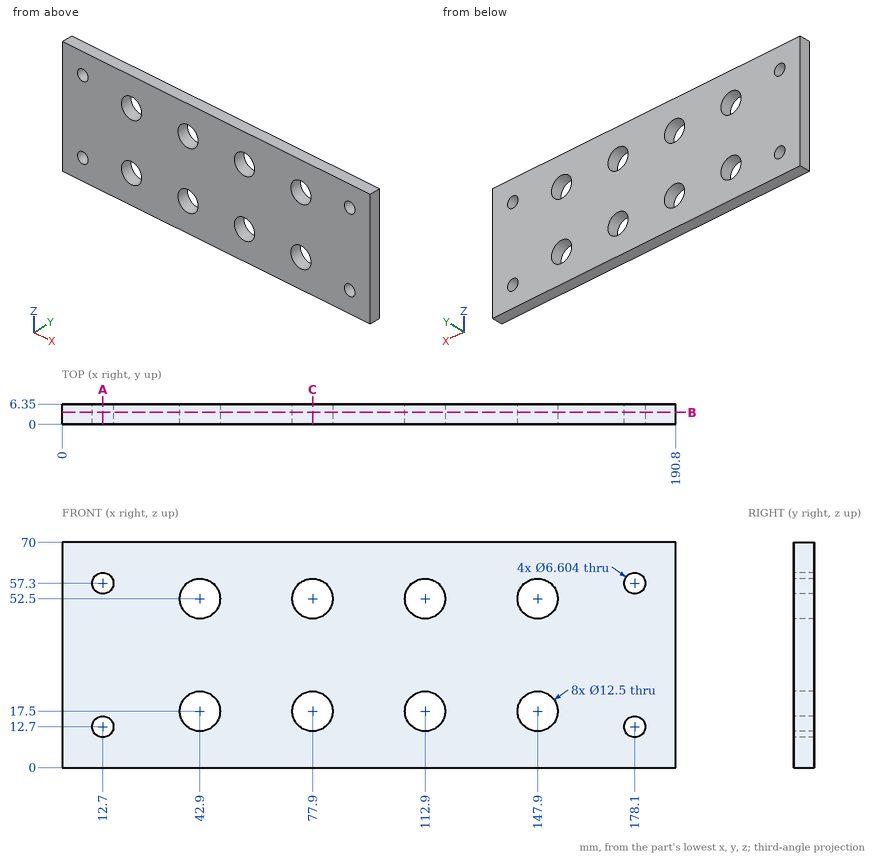
Geometry check sheet. Reference: drawing and pictorial views, mm from the part's lowest x, y, z. Round coordinates to 2 decimals unless told otherwise and drop trailing zeros. Loops run counter-clockwise (first coordinate to the right, second up) from the corner with the lowest first, then second, coordinate; pieces in that order, holes last. Notation, with made-up numbers: (86.5, 50) - (99.5, 50) arc R24 ccw to (99.5, 87) - close; hole circle Ø7 at (52.25, 38). An arc over 180 degrees is marked (long way). Write item = value, one per line. Start each with the question number.
Q1. Depth check by flat-ended pin: P1, Ø7.5, axis at x = 42.9, z = 17.5, coming from the -Y side. Enter the tip coordinate at first touch or a pass-through.
Q2. Section check C-C (x = 77.9). Record the boundary of the cut face in (y, z).
Q3. Thickness scan on L1, parallel to Z at x = 43.5, y = 0.5; L2, parallel to Z at x = 149.5, y = 5.5; L3, parallel to X at y = 4, z = 22.5. Record the ranges inside material, lowest first.
Q4. Section check A-A (x = 12.7). Record the boundary of the cut face in (y, z).
Q5. Section check B-B (y = 3.75). Count the separate pieces of the cut face and the enclosed holes in it, plus the area to 3 significant figures.
Derived:
q1.P1 = through
q2.outline = (0, 0) - (6.35, 0) - (6.35, 11.25) - (0, 11.25) - close; (0, 23.75) - (6.35, 23.75) - (6.35, 46.25) - (0, 46.25) - close; (0, 58.75) - (6.35, 58.75) - (6.35, 70) - (0, 70) - close
q3.L1 = 0 to 11.28, 23.72 to 46.28, 58.72 to 70
q3.L2 = 0 to 11.46, 23.54 to 46.46, 58.54 to 70
q3.L3 = 0 to 39.15, 46.65 to 74.15, 81.65 to 109.15, 116.65 to 144.15, 151.65 to 190.8
q4.outline = (0, 0) - (6.35, 0) - (6.35, 9.4) - (0, 9.4) - close; (0, 16) - (6.35, 16) - (6.35, 54) - (0, 54) - close; (0, 60.6) - (6.35, 60.6) - (6.35, 70) - (0, 70) - close
q5.separate_pieces = 1
q5.enclosed_holes = 12
q5.area = 12,200 mm^2
